from build123d import *

# Parameters (mm, degrees)
SKETCH_1_R          = 3.025
SKETCH_1_R_2        = 2.025
EXTRUDE_1_DEPTH     = 4
SKETCH_2_W          = 79
SKETCH_2_H          = 30
CUT_EXTRUDE_1_DEPTH = 4
FILLET_1_R          = 4
CHAMFER_1_SIZE      = 8
FILLET_2_R          = 4


with BuildPart() as part:
    # 草图1 → 凸台-拉伸1 (new body)
    with BuildSketch(Plane.XY):
        Polygon((-71.051486421, 22), (-118, -41.5), (-148, -41.5), (-148, -61.5), (-107.914189298, -61.5), (-77.231302471, -20), (77.231302471, -20), (107.914189298, -61.5), (148, -61.5), (148, -41.5), (118, -41.5), (71.051486421, 22), align=None)
        with Locations((-97.615651235, -30.75)):
            Circle(SKETCH_1_R, mode=Mode.SUBTRACT)
        with Locations((97.615651235, -30.75)):
            Circle(SKETCH_1_R, mode=Mode.SUBTRACT)
        with Locations((-65, -10)):
            Circle(SKETCH_1_R_2, mode=Mode.SUBTRACT)
        with Locations((-47.5, -8.5)):
            Circle(SKETCH_1_R_2, mode=Mode.SUBTRACT)
        with Locations((-65, 10)):
            Circle(SKETCH_1_R_2, mode=Mode.SUBTRACT)
        with Locations((-47.5, 16.5)):
            Circle(SKETCH_1_R_2, mode=Mode.SUBTRACT)
        with Locations((65, -10)):
            Circle(SKETCH_1_R_2, mode=Mode.SUBTRACT)
        with Locations((47.5, -8.5)):
            Circle(SKETCH_1_R_2, mode=Mode.SUBTRACT)
        with Locations((65, 10)):
            Circle(SKETCH_1_R_2, mode=Mode.SUBTRACT)
        with Locations((47.5, 16.5)):
            Circle(SKETCH_1_R_2, mode=Mode.SUBTRACT)
        with Locations((-123, -51.5)):
            Circle(SKETCH_1_R_2, mode=Mode.SUBTRACT)
        with Locations((-143, -51.5)):
            Circle(SKETCH_1_R_2, mode=Mode.SUBTRACT)
        with Locations((-133, -51.5)):
            Circle(SKETCH_1_R, mode=Mode.SUBTRACT)
        with Locations((143, -51.5)):
            Circle(SKETCH_1_R_2, mode=Mode.SUBTRACT)
        with Locations((123, -51.5)):
            Circle(SKETCH_1_R_2, mode=Mode.SUBTRACT)
        with Locations((133, -51.5)):
            Circle(SKETCH_1_R, mode=Mode.SUBTRACT)
    extrude(amount=EXTRUDE_1_DEPTH)

    # 草图2 → 切除-拉伸1 (cut)
    with BuildSketch(Plane.XY.offset(4)):
        with Locations((0, 1)):
            Rectangle(SKETCH_2_W, SKETCH_2_H)
    extrude(amount=-CUT_EXTRUDE_1_DEPTH, mode=Mode.SUBTRACT)

    # 圆角1
    fillet_1_edges = [part.edges().sort_by_distance(p)[0] for p in [
        (-148, -61.5, 2),
        (-148, -41.5, 2),
        (-118, -41.5, 2),
        (-71.051486421, 22, 2),
        (71.051486421, 22, 2),
        (118, -41.5, 2),
        (148, -41.5, 2),
        (148, -61.5, 2),
        (107.914189298, -61.5, 2),
        (77.231302471, -20, 2),
        (-77.231302471, -20, 2),
        (-107.914189298, -61.5, 2),
    ]]
    fillet(fillet_1_edges, radius=FILLET_1_R)

    # 倒角1
    chamfer_1_edges = [part.edges().sort_by_distance(p)[0] for p in [
        (39.5, 16, 2),
        (39.5, -14, 2),
        (-39.5, -14, 2),
        (-39.5, 16, 2),
    ]]
    chamfer(chamfer_1_edges, length=CHAMFER_1_SIZE)

    # 圆角2
    fillet_2_edges = [part.edges().sort_by_distance(p)[0] for p in [
        (39.5, 8, 2),
        (39.5, -6, 2),
        (-31.5, -14, 2),
        (31.5, -14, 2),
        (-31.5, 16, 2),
        (31.5, 16, 2),
        (-39.5, -6, 2),
        (-39.5, 8, 2),
    ]]
    fillet(fillet_2_edges, radius=FILLET_2_R)


solid = part.part
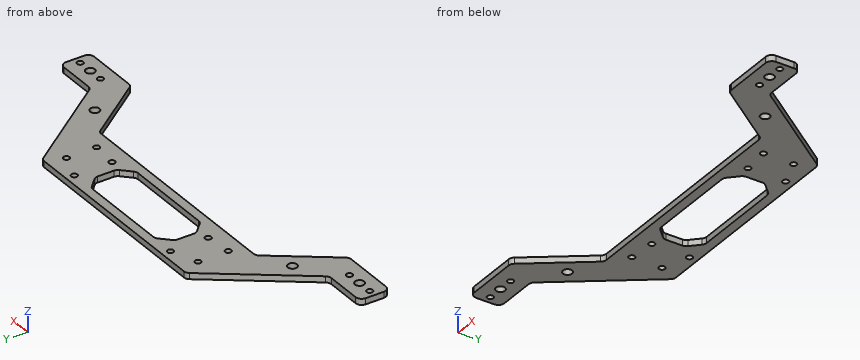
Source: CAD feature listing. Evaluate the final solid. Frame: model axes, mm. Round coordinates to 2 decimals unless told otherwise and drop trailing zeros. Order: outer loops, then holes, each group sorted by start corner. A loop starts at its lowest first (then second) coordinate and runs counter-clockwise, first axis right, second up. Notation, with made-up numbers: (-28, 18.25) - (22, 18.25) arc R35 ccw to (22, 53.25) - close; hole circle Ø6 at (56.5, 7). An arc over 180 degrees is marked (long way). Use a Markdown table: item, result. Add a question column.
1. Section query A-A (x = 3). Return the cut outline in (y, z).
2. Section query B-B (z = 1.2). Give the number of separate pieces and of enclosed holes in the cut face, then the cut area to 3 significant figures.
3. Section query C-C (y = -30.75). Return the cut outline in (x, z).
4. Section query D-D (x = -133). Return the cut outline in (y, z) (3 decimals).
5. Line query: probe 1 along Y at (x, z) = (-47.5, 2.4) (3 decimals); probe 2 along Y at (x, z) = (65, 1.6) (3 decimals); probe 3 along Y at (x, z) = (132.5, 1.35). Output: solid intervals per line, ascending.
6. First-contact query: pin 1 (1.5 mm diameter, centred on y = -38.5, z = 1, fed in from +X); pin 2 (2.5 mm diameter, centred on x = -65, y = 10, fed in from +Z); pin 3 (2 mm diameter, centred on x = -2.5, z = 2, fed in from -Y); pin 4 (1.2 mm diameter, centred on y = 1.5, z = 1.5, fed in from +X). Flat tips, straight axial feed; report the tip coordinate or a pass-through.
Derived:
| question | item | result |
|---|---|---|
| 1 | outline | (-20, 0) - (-14, 0) - (-14, 4) - (-20, 4) - close; (16, 0) - (22, 0) - (22, 4) - (16, 4) - close |
| 2 | separate pieces | 1 |
| 2 | enclosed holes | 17 |
| 2 | area | 7,720 mm2 |
| 3 | outline | (-110.05, 0) - (-100.64, 0) - (-100.64, 4) - (-110.05, 4) - close; (-94.59, 0) - (-85.18, 0) - (-85.18, 4) - (-94.59, 4) - close; (85.18, 0) - (94.59, 0) - (94.59, 4) - (85.18, 4) - close; (100.64, 0) - (110.05, 0) - (110.05, 4) - (100.64, 4) - close |
| 4 | outline | (-61.5, 0) - (-54.525, 0) - (-54.525, 4) - (-61.5, 4) - close; (-48.475, 0) - (-41.5, 0) - (-41.5, 4) - (-48.475, 4) - close |
| 5 | probe 1 | -20 to -10.525, -6.475 to 14.475, 18.525 to 22 |
| 5 | probe 2 | -20 to -12.025, -7.975 to 7.975, 12.025 to 22 |
| 5 | probe 3 | -61.5 to -54.48, -48.52 to -41.5 |
| 6 | pin 1 | x = 116.34 |
| 6 | pin 2 | through |
| 6 | pin 3 | y = -20 |
| 6 | pin 4 | x = 86.65 |
